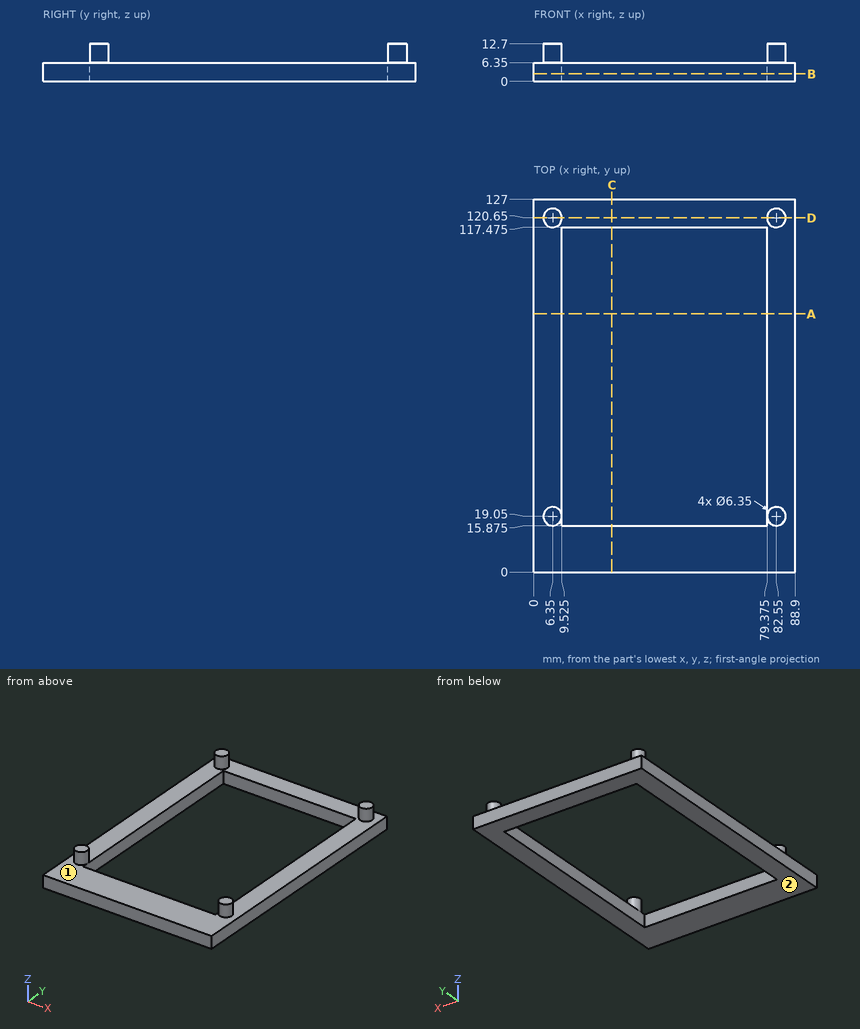
Here's the drawing with two shaded views (mm, measured from the low corner). I have some questions. A direction names the side the tool comes from. Coordinates: 2 decimals unless noted, no trailing zeros. Order: outer loops, then holes, each group sorted by start corner. A loop starts at its lowest first (then second) coordinate and runs counter-clockwise, first axis right, second up. Notation, with made-up numbers: M -39,-15.5 L -21,-15.5 A18 ccw -21,7.5 Z; hole C 35,-15.5 d10. An arc over 180 degrees is marked long. Answer as CSV lines item,"result".
Item 1: If I drill on line 1 (X direction, y = 98, z = 4.5) (3 decimals); line 2 (Y direction, x = 18, z = 4) (3 decimals); line 3 (Z direction, x = 57, y = 118), over which ranges is the centre line in solid material (lowest first)?
Results found:
line 1,"0 to 9.525, 79.375 to 88.9"
line 2,"0 to 15.875, 117.475 to 127"
line 3,"0 to 6.35"
Item 2: Imagine slicing it at D-D on y = 120.65. Write out the boundary of the cut face in (x, z) (3 decimals).
Results found:
outline,"M 0,0 L 88.9,0 L 88.9,6.35 L 85.725,6.35 L 85.725,12.7 L 79.375,12.7 L 79.375,6.35 L 9.525,6.35 L 9.525,12.7 L 3.175,12.7 L 3.175,6.35 L 0,6.35 Z"
Item 3: Imagine slicing it at A-A on y = 88. Write out the boundary of the cut face in (x, z) (3 decimals), plus the area to 3 significant figures.
Results found:
outline,"M 0,0 L 9.525,0 L 9.525,6.35 L 0,6.35 Z; M 79.375,0 L 88.9,0 L 88.9,6.35 L 79.375,6.35 Z"
area,"121 mm2"
Item 4: On a 3-axis mill with a long thin cutter (end or side, diameter ignored), from which of +Z, -Z, +X, -X, +Y, -Y can I reach the whole of each face in a straight line? I mean the marked faces 1 and 2. Say none if no direction works.
Results found:
face 1,"+Z"
face 2,"-Z, +X, -X, +Y, -Y"
Item 5: For pin 1 (8 mm diameter, centred on x = 29.5, y = 13.5, fed in from +Z); pin 2 (3 mm diameter, centred on x = 74.5, z = 8.5, fed in from +Y), each with a flat end and sliding along its axis, tell me the tip position at first contact or that it passes through.
Results found:
pin 1,"z = 6.35"
pin 2,"through"
Item 6: Imagine slicing it at C-C on x = 26.5. Write out the boundary of the cut face in (y, z) (3 decimals).
Results found:
outline,"M 0,0 L 15.875,0 L 15.875,6.35 L 0,6.35 Z; M 117.475,0 L 127,0 L 127,6.35 L 117.475,6.35 Z"
Item 7: Imagine slicing it at B-B on z = 2.5. Write out the boundary of the cut face in (x, y) (3 decimals).
Results found:
outline,"M 0,0 L 88.9,0 L 88.9,127 L 0,127 Z; hole M 9.525,15.875 L 79.375,15.875 L 79.375,117.475 L 9.525,117.475 Z"
